Design review of the part built by this model. Coordinates are the model's own, in mm. A direction names the side the tool comes from. Give positions to 0.01 mm unless a question says otherwise; leave off trailing zeros. Loops run counter-clockwise (first coordinate to the right, second up) from the corner with the lowest first, then second, coordinate; pieces in that order, holes last. Notation, with made-up numbers: M -8.75,30 L 40.25,30 A20 cw 40.25,53 Z; hole C 3.25,-35 d4. An arc over 180 degrees is marked long. Use a Markdown table: item, result. Add a question column.
(1) Insertion check: pin 1 Ø5 at (y, z) = (25, 96) entering from -X (1 decimal); pin 2 Ø3 at (x, y) = (3.5, 13.5) entering from +Z; pin 3 Ø1 at (x, z) = (4, 86) entering from -Y; pin 4 Ø1.5 at (x, y) = (2, 24) entering from -Z. Each pin has a flat end and moves straight along its axis. Give the tip position at first contact, or say it passes through.
(2) Add section C-C, the plane z = 63. Give the boundary of the cut face in (x, y).
(3) For probe 1 along Y at (x, z) = (4.7, 37.5); probe 2 along Z at (x, y) = (0.45, 29); probe 3 along Y at (x, z) = (3.4, 62), list the stretches that pass through material, from the lowest coordinate up.
(4) For faces 5 (the face through (2, 0, 27)), 6 (the face through (2.46, 16.59, -0.34)), list the 3-axis set-ups (+Z, -Z, +X, -X, +Y, -Y) from which the entire face can be reached by the end or side of a thin tool; tool diameter is ignored.
(5) Draft analysis for pull direction Y (two halves, no side actions). For faces 1 (the face through (2.535, 49.449, 0.284)), 2 (the face through (4.5, 25.1, 99)), 3 (the face through (2, 7, 60)), 4 (the face through (5, 8, 58)), state which applies: pulls with the +Y half, pulls with the -Y half, needs draft (parallel to the pull), parting line crosses it, or undercut.
(6) Add section D-D, the plane y = 25. Give the boundary of the cut face in (x, z), then the cut area to 3 significant figures.
(7) Add section B-B, the plane x = 1.2. Give the boundary of the cut face in (y, z), then the cut area to 3 significant figures.
(8) Add section A-A, the plane z = 21. Give the boundary of the cut face in (x, y).
Autodesk Inventor part; units mm, degrees
ref_plane "YZ Plane" through (0, 0, 0) normal (1, 0, 0) x (0, 1, 0)
ref_plane "XZ Plane" through (0, 0, 0) normal (0, 1, 0) x (-1, 0, 0)
ref_plane "XY Plane" through (0, 0, 0) normal (0, 0, 1) x (1, 0, 0)
sketch "Sketch1" plane through (0, 0, 0) normal (1, 0, 0) x (0, 1, 0)
  line L0 (0, 0) -> (50, 0)
  line L1 (50, 0) -> (50, 110)
  line L2 (50, 110) -> (0, 110)
  line L3 (0, 110) -> (0, 0)
  line L4 (50, 0) -> (0, -28.8675)
  line L5 (0, -28.8675) -> (0, 0)
  dimension "d0" = 110
  dimension "d1" = 50
  dimension "d68" = 60
extrude "Extrusion1" add sketch "Sketch1" along normal blind 5
fillet "Fillet1" radius 4 2 edges at (2.5, 50, 0) (2.5, 0, -28.8675)
sketch "Sketch2" plane through (5, 0, 0) normal (1, 0, 0) x (0, 0, -1)
  line L0 (-2.3094, 50) -> (-110, 50)
  line L1 (-110, 50) -> (-110, 0)
  line L2 (-110, 33.9915) -> (-75, 50)
  line L3 (-110, 16.0085) -> (-75, 0)
  line L4 (-110, 50) -> (-56.045, 50)
  line L5 (-56.045, 50) -> (-56.045, 0)
  line L6 (-56.045, 0) -> (-110, 0)
  line L7 (-110, 0) -> (-110, 50)
  line L8 (-110, 33.9915) -> (-110, 16.0085)
  line L9 (-110, 50) -> (-110, 0)
  line L10 (-110, 0) -> (-75, 0)
  circle A0 centre (-96, 25) radius 14
  circle A1 centre (-96, 25) radius 8.05
  line L11 (-96, 25) -> (-90.3078, 19.3078)
  line L12 (-96, 25) -> (-87.95, 25) construction
  circle A2 centre (-90.3078, 19.3078) radius 1.5
  circle A3 centre (-90.3078, 30.6922) radius 1.5
  circle A4 centre (-101.6922, 30.6922) radius 1.5
  circle A5 centre (-101.6922, 19.3078) radius 1.5
  circle A6 centre (-96, 25) radius 3
  point P0 (0, 0)
  point P1 (-110, 0)
  point P2 (-75, 0)
  point P3 (-110, 25)
  point P4 (-101.8232, 37.7315)
  point P5 (-101.8232, 12.2685)
  dimension "d84" = 16.1
  dimension "d13" = 35
  dimension "d82" = 28
  dimension "d83" = 25
  dimension "d86" = 45
  dimension "d87" = 3
  dimension "d90" = 360
  dimension "d97" = 6
extrude "Extrusion2" cut sketch "Sketch2" against normal blind 5 contours L2 L1 L0 | A0 L1 L2 | L6 L1 L3 | A0 L3 L1 | A6
fillet "Fillet3" radius 4 1 edges at (2.5, 50, 75)
chamfer "Chamfer2" distance 4 angle 45 1 edges at (0, 25, 99)
sketch "Sketch7" plane through (0, 0, 0) normal (-1, 0, 0) x (0, 0, 1)
  circle A0 centre (63, 43) radius 3
  circle A1 centre (63, 7) radius 3
  circle A2 centre (-14, 7) radius 3
  line L0 (74.1286, 0) -> (-21.9393, 0)
  line L1 (2.3094, 50) -> (74.1286, 50)
  point P0 (0, 0)
  dimension "d101" = 14
  dimension "d102" = 63
  dimension "d103" = 7
  dimension "d104" = 7
  dimension "d105" = 6
extrude "Extrusion7" cut sketch "Sketch7" against normal blind 7
sketch "Sketch8" plane through (0, 0, 0) normal (-1, 0, 0) x (0, 0, 1)
  line L0 (4.6188, 42) -> (48.7321, 42)
  line L1 (48.7321, 42) -> (48.7321, 8)
  line L2 (48.7321, 8) -> (4.6188, 8)
  line L3 (4.6188, 8) -> (4.6188, 42)
  line L4 (4.6188, 42) -> (-5.1962, 25)
  line L5 (-5.1962, 25) -> (4.6188, 8)
  line L6 (48.7321, 8) -> (78.1769, 25)
  line L7 (78.1769, 25) -> (48.7321, 42)
  line L8 (-25.4034, 6) -> (-1.1547, 48)
  line L9 (2.3094, 50) -> (74.1286, 50)
  line L10 (74.1286, 0) -> (-21.9393, 0)
  circle A0 centre (63, 43) radius 3
  point P0 (0, 0)
  dimension "d108" = 8
  dimension "d109" = 8
  dimension "d110" = 8
  dimension "d111" = 8
extrude "Extrusion8" cut sketch "Sketch8" against normal blind 7 contours L0 L1 L2 L3 | L3 L5 L4 | L7 L6 L1
fillet "Fillet5" radius 4 6 edges at (2.5, 42, 4.6188) (2.5, 25, -5.1962) (2.5, 8, 4.6188) (2.5, 8, 48.7321) (2.5, 25, 78.1769) (2.5, 42, 48.7321)
properties part number "frame_side"
Established:
| question | item | result |
|---|---|---|
| 1 | pin 1 | through |
| 1 | pin 2 | z = 105.8 |
| 1 | pin 3 | y = 4.8 |
| 1 | pin 4 | z = -15.44 |
| 2 | outline | M 0,0 L 5,0 L 5,4 L 0,4 Z; M 0,10 L 5,10 L 5,16.24 L 0,16.24 Z; M 0,33.76 L 5,33.76 L 5,40 L 0,40 Z; M 0,46 L 5,46 L 5,50 L 0,50 Z |
| 3 | probe 1 | 0 to 8, 42 to 50 |
| 3 | probe 2 | -12.12 to -2.89, 71.25 to 90.81, 101.19 to 109.42 |
| 3 | probe 3 | 0 to 4.17, 9.83 to 15.66, 34.34 to 40.17, 45.83 to 50 |
| 4 | face 5 | +Z, -Z, +X, -X, -Y |
| 4 | face 6 | +X, -X |
| 5 | face 1 | pulls with the +Y half |
| 5 | face 2 | undercut |
| 5 | face 3 | undercut |
| 5 | face 4 | needs draft |
| 6 | outline | M 0,-14.43 L 5,-14.43 L 5,-4.58 L 0,-4.58 Z; M 0,74.18 L 5,74.18 L 5,93 L 4,93 L 0,89 Z; M 0,103 L 4,99 L 5,99 L 5,110 L 0,110 Z |
| 6 | area | 182 mm^2 |
| 7 | outline | M 0,-21.94 A4 ccw 6,-25.4 L 48,-1.15 A4 ccw 50,2.31 L 50,74.13 A4 ccw 49.64,75.79 L 37.73,101.82 A14 ccw 12.27,101.82 L 0,75 Z; hole C 7,-14 d6; hole C 7,63 d6; hole M 8,6.93 A4 ccw 10,3.46 L 23,-4.04 A4 ccw 27,-4.04 L 40,3.46 A4 ccw 42,6.93 L 42,47.66 A4 ccw 41.46,49.66 L 28.46,72.18 A4 ccw 21.54,72.18 L 8.54,49.66 A4 ccw 8,47.66 Z; hole C 25,96 d11.6; hole C 43,63 d6 |
| 7 | area | 3,280 mm^2 |
| 8 | outline | M 0,0 L 5,0 L 5,8 L 0,8 Z; M 0,42 L 5,42 L 5,50 L 0,50 Z |
